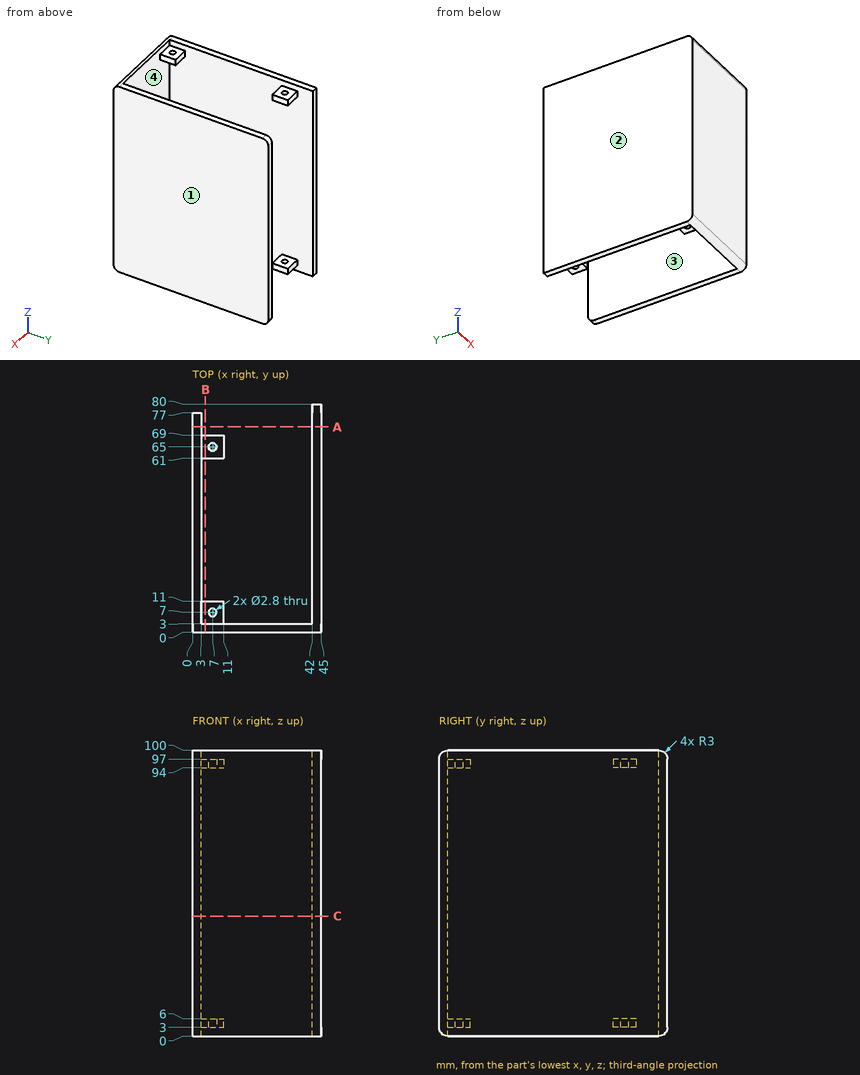
Design review of the part shown in the three views and the two pictorial views. Dimensions are in mm from the part's minimum x, y and z. Give positions to 0.01 mm unless a question says otherwise; leave off trailing zeros. Loops run counter-clockwise (first coordinate to the right, second up) from the corner with the lowest first, then second, coordinate; pieces in that order, holes last. Notation, with made-up numbers: (78.25, 22) -> (83.25, 22) arc R24 cw to (83.25, 40) -> close; hole circle Ø9 at (65, -40). An arc over 180 degrees is marked (long way). One line per question, with ' | ' between items.
1) Insertion check: pin 1 Ø19.5 at (x, z) = (30.5, 26) entering from +Y; pin 2 Ø0.9 at (x, z) = (5, 96) entering from +Y; pin 3 Ø1 at (y, z) = (36.5, 77.5) entering from -X; pin 4 Ø3.5 at (x, y) = (7, 7) entering from -Z. Each pin has a flat end and moves straight along its axis. Give the tip position at first contact, or say it passes through.
Resolved:
pin 1: stops at y = 3 | pin 2: stops at y = 69 | pin 3: stops at x = 0 | pin 4: stops at z = 3
2) To check wall thickness, follow probe 1 along Y at (x, z) = (7, 95); probe 2 along X at (y, z) = (54.5, 41); probe 3 along X at (y, z) = (65, 4.55). State the ranges of each line that lie inside material, in increasing order.
Resolved:
probe 1: y = 0 to 5.6, 8.4 to 11, 61 to 63.6, 66.4 to 69 | probe 2: x = 0 to 3, 42 to 45 | probe 3: x = 0 to 5.6, 8.4 to 11, 42 to 45
3) We need section B-B (x = 4.5). Write out the cut boundary in (y, z), plus the area to 3 significant figures.
Resolved:
outline: (0, 3) arc R3 ccw to (3, 0) -> (3, 3) -> (11, 3) -> (11, 6) -> (3, 6) -> (3, 94) -> (11, 94) -> (11, 97) -> (3, 97) -> (3, 100) arc R3 ccw to (0, 97) -> close; (61, 3) -> (69, 3) -> (69, 6) -> (61, 6) -> close; (61, 94) -> (69, 94) -> (69, 97) -> (61, 97) -> close | area: 392 mm2
4) We need section C-C (z = 42). Write out the cut boundary in (x, y), plus the area to 3 significant figures.
Resolved:
outline: (0, 0) -> (45, 0) -> (45, 80) -> (42, 80) -> (42, 3) -> (3, 3) -> (3, 77) -> (0, 77) -> close | area: 588 mm2
5) We need section A-A (y = 72). Write out the cut boundary in (x, z).
Resolved:
outline: (0, 0) -> (3, 0) -> (3, 100) -> (0, 100) -> close; (42, 0) -> (45, 0) -> (45, 100) -> (42, 100) -> close
6) The part is to be moulded in two halves that separate along X. For the marked faces 1, 2, 3 and 4, say which applies: +X half, -X half, draft (parallel to the pull), parting line (faces both ways), or undercut.
Resolved:
face 1: +X half | face 2: -X half | face 3: undercut | face 4: undercut
